from build123d import *

# Parameters (mm, degrees)
F0_R     = 3.175
F1_DEPTH = 15.875
F2_W     = 76.2
F2_H     = 6.604
F3_DEPTH = 25.4


# Not quite as in the source:
# - a length typed as a fraction of an inch, garbled in the dataset ("3 / 203.2 mm" for 3/8 in), is restored


with BuildPart() as f1:
    # F0 (on Front) → F1 (new body)
    with BuildSketch(Plane.XZ):
        with BuildLine():
            Line((127, 9.525), (0, 9.525))
            ThreePointArc((0, 9.525), (-9.3531345836, 1.801249139), (-3.5374961923, -8.8437404807))
            Line((-3.5374961923, -8.8437404807), (28.2125038077, -21.5437404807))
            ThreePointArc((28.2125038077, -21.5437404807), (34.4639700258, -21.8301693138), (39.543916522, -18.1754442969))
            ThreePointArc((39.543916522, -18.1754442969), (54.4695569537, -6.6633605399), (73.291331011, -5.641775468))
            ThreePointArc((73.291331011, -5.641775468), (101.4455517982, -8.4127099235), (129.1718279101, -2.792048142))
            ThreePointArc((129.1718279101, -2.792048142), (133.2535292316, 4.2776659282), (127, 9.525))
        make_face()
        with Locations((31.75, -12.7)):
            Circle(F0_R, mode=Mode.SUBTRACT)
        Circle(F0_R, mode=Mode.SUBTRACT)
    extrude(amount=F1_DEPTH)

    # F2 (on face) → F3 (cut)
    with BuildSketch(Plane(origin=(-3.5374961923, 0, -8.8437404807), x_dir=(0.9284766909, 0, -0.3713906764), z_dir=(-0.3713906764, 0, -0.9284766909))):
        with Locations((17.0978982627, 7.9375)):
            Rectangle(F2_W, F2_H)
    extrude(amount=-F3_DEPTH, mode=Mode.SUBTRACT)


solid = f1.part
Source: CAD feature listing. Evaluate the final solid. Frame: model axes, mm. A direction names the side the tool comes from. Give positions to 0.01 mm unless a question says otherwise; leave off trailing zeros. Order: outer loops, then holes, each group sorted by start corner. A loop starts at its lowest first (then second) coordinate and runs counter-clockwise, first axis right, second up. Notation, with made-up numbers: (-18, -37) -> (29, -37) arc R18 cw to (29, -6) -> close; hole circle Ø8 at (-28, -5.75). An arc over 180 degrees is marked (long way). Use a Markdown table: item, result.
1) Mould query, pull axis X, two halves, no side actions, for faces 1 (the cylindrical face through (34.378, -13.525, -21.855)), 2 (the cylindrical face through (-9.317, -13.525, 1.982)), 3 (the cylindrical face through (31.06, -13.52, -15.8)). Classes: +X half, -X half, draft (parallel to the pull), parting line (faces both ways), or undercut.
Answer list:
| item | result |
|---|---|
| face 1 | parting line |
| face 2 | -X half |
| face 3 | undercut |
2) Section query D-D, the plane x = 51. Return the cut outline in (y, z) (1 decimal), then the cut area to 3 significant figures.
Answer list:
| item | result |
|---|---|
| outline | (-15.9, -8.2) -> (-11.2, -8.2) -> (-11.2, -3.3) -> (-4.6, -3.3) -> (-4.6, -8.2) -> (0, -8.2) -> (0, 9.5) -> (-15.9, 9.5) -> close |
| area | 249 mm² |
3) Reachability of faces 4 (the flat face through (64, -8, 9.525)), 5 (the flat face through (22, -4.636, -6)) from +Z, -Z, +X, -X, +Y, -Y: full face, straight path, thin tool, end or side. Return the list, or none.
Answer list:
| item | result |
|---|---|
| face 4 | +Z, +X, -X, +Y, -Y |
| face 5 | -Z, -X |
4) Contact query for flat-ended pins moving along their axis: P1, Ø6, axis at x = 46, z = 3, coming from the +Y side; P2, Ø5, axis at x = 0, z = 0, coming from the +Y side. Output: stop coordinate, or through.
Answer list:
| item | result |
|---|---|
| P1 | y = 0 |
| P2 | through |
5) Section query C-C, the plane x = 31.75. Return the cut outline in (y, z) (1 decimal), then the cut area to 3 significant figures.
Answer list:
| item | result |
|---|---|
| outline | (-15.9, -22.2) -> (-11.2, -22.2) -> (-11.2, -15.9) -> (-15.9, -15.9) -> close; (-15.9, -9.5) -> (-11.2, -9.5) -> (-11.2, 4.4) -> (-4.6, 4.4) -> (-4.6, -9.5) -> (0, -9.5) -> (0, 9.5) -> (-15.9, 9.5) -> close; (-4.6, -22.2) -> (0, -22.2) -> (0, -15.9) -> (-4.6, -15.9) -> close |
| area | 269 mm² |
6) Section query B-B, the plane y = -3. Count the separate pieces of the cut face and the enclosed holes in it, then the cut area to 3 significant figures.
Answer list:
| item | result |
|---|---|
| separate pieces | 1 |
| enclosed holes | 2 |
| area | 2,690 mm² |
7) Ray query, line 1 along Y through (x, z) = (21.5, -1.5) (1 decimal); line 2 along Z through (x, y) = (74, -9) (3 decimals); line 3 along Z through (x, y) = (31.75, -2.6) (3 decimals). Return the intervals inside material, ascending. Write a range as [from, to].
Answer list:
| item | result |
|---|---|
| line 1 | [-15.9, -11.2], [-4.6, 0] |
| line 2 | [-5.818, 9.525] |
| line 3 | [-22.225, -15.875], [-9.525, 9.525] |
8) Section query A-A, the plane z = -7. Return the cut outline in (x, y) (1 decimal).
Answer list:
| item | result |
|---|---|
| outline | (-6.5, -15.9) -> (53.6, -15.9) -> (53.6, -11.2) -> (-6.5, -11.2) -> close; (-6.5, -4.6) -> (53.6, -4.6) -> (53.6, 0) -> (-6.5, 0) -> close; (79.6, -15.9) -> (113.6, -15.9) -> (113.6, 0) -> (79.6, 0) -> close |
